Read the model definition and answer for the solid it produces. Units are mm, in the model's axes. Give positions to 0.01 mm unless a question says otherwise; leave off trailing zeros. Order: outer loops, then holes, each group sorted by start corner. A loop starts at its lowest first (then second) coordinate and runs counter-clockwise, first axis right, second up.
Item 1: A cutting plane is placed at C-C (z = -4.75). Write down the section's boundary in (x, y), plus the area to 3 significant figures.
Item 2: Find the intervals of material crossed by line 1 along Y through (x, z) = (7.45, -2.75); line 2 along Y through (x, z) = (7.45, 6.75); line 3 along Z through (x, y) = (7.35, 4.5), in increasing order.
Item 3: The mould has two halves that part along Y. Classify faces 1 (the face through (7.446, 4.859, 6.667)), 2 (the face through (7.45, -2.38, -3.17)), 3 (the face through (7.45, -3.75, 1.28)): +Y half, -Y half, draft (parallel to the pull), parting line (faces both ways), or undercut.
Item 4: A cutting plane is placed at B-B (y = 4.5). Write down the section's boundary in (x, z), plus the area to 3 significant figures.
Item 5: A cutting plane is placed at D-D (y = 1.25). Write down the section's boundary in (x, z), plus the area to 3 significant figures.
from build123d import *

# Parameters (mm, degrees)
ESTRUSIONE_ESTRUSIONE1_DEPTH = 0.5


with BuildPart() as part:
    # Schizzo1 → Estrusione-Estrusione1 (new body)
    with BuildSketch(Plane(origin=(7.692307692, 0, 0), x_dir=(0, 0, -1), z_dir=(1, 0, 0))):
        with BuildLine():
            Line((-6.113475279, -5.539667861), (-5.372640914, -4.868367801))
            ThreePointArc((-5.372640914, -4.868367801), (-1.224247655, -3.767846854), (1.485003008, -7.096551381))
            Line((1.485003008, -7.096551381), (1.689770324, -8.075096052))
            ThreePointArc((1.689770324, -8.075096052), (2.549390204, -7.846216259), (3.379369462, -7.526112014))
            Line((3.379369462, -7.526112014), (2.969855574, -6.614093536))
            ThreePointArc((2.969855574, -6.614093536), (3.205121972, -2.32865742), (7.2081126, -0.780633191))
            Line((7.2081126, -0.780633191), (8.202040467, -0.888274834))
            ThreePointArc((8.202040467, -0.888274834), (8.25, 0), (8.202040467, 0.888274834))
            Line((8.202040467, 0.888274834), (7.2081126, 0.780633191))
            ThreePointArc((7.2081126, 0.780633191), (3.205121972, 2.32865742), (2.969855574, 6.614093536))
            Line((2.969855574, 6.614093536), (3.379369462, 7.526112014))
            ThreePointArc((3.379369462, 7.526112014), (2.549390204, 7.846216259), (1.689770324, 8.075096052))
            Line((1.689770324, 8.075096052), (1.485003008, 7.096551381))
            ThreePointArc((1.485003008, 7.096551381), (-1.224247655, 3.767846854), (-5.372640914, 4.868367801))
            Line((-5.372640914, 4.868367801), (-6.113475279, 5.539667861))
            ThreePointArc((-6.113475279, 5.539667861), (-6.674390204, 4.849228331), (-7.157704974, 4.102408989))
            Line((-7.157704974, 4.102408989), (-6.290330268, 3.605276765))
            ThreePointArc((-6.290330268, 3.605276765), (-3.961748634, 0), (-6.290330268, -3.605276765))
            Line((-6.290330268, -3.605276765), (-7.157704974, -4.102408989))
            ThreePointArc((-7.157704974, -4.102408989), (-6.674390204, -4.849228331), (-6.113475279, -5.539667861))
        make_face()
    extrude(amount=-ESTRUSIONE_ESTRUSIONE1_DEPTH)


solid = part.part
Response values:
1. outline: (7.19, -1.06) - (7.69, -1.06) - (7.69, 1.06) - (7.19, 1.06) - close
1. area: 1.06 mm2
2. line 1: y = -7.78 to -6.17, -3.14 to 3.14, 6.17 to 7.78
2. line 2: y = -4.74 to -3.87, 3.87 to 4.74
2. line 3: z = -2.45 to -0.1, 4.99 to 6.91
3. face 1: +Y half
3. face 2: undercut
3. face 3: -Y half
4. outline: (7.19, -2.45) - (7.69, -2.45) - (7.69, -0.1) - (7.19, -0.1) - close; (7.19, 4.99) - (7.69, 4.99) - (7.69, 6.91) - (7.19, 6.91) - close
4. area: 2.14 mm2
5. outline: (7.19, -4.39) - (7.69, -4.39) - (7.69, 4.16) - (7.19, 4.16) - close
5. area: 4.28 mm2
